Design review of the part built by this model. Coordinates are the model's own, in mm. Coordinates: 2 decimals unless noted, no trailing zeros. Write each loop counter-clockwise with the first axis right and the second up, starting at its lowest first coordinate (ties: lowest second). Pieces come first, ordered by that corner, then holes. Notation, with made-up numbers: (-14.75, 78.5) - (12.25, 78.5) arc R34 cw to (12.25, 111.5) - close; hole circle Ø8 at (61.5, -35.5). An arc over 180 degrees is marked (long way). Use a Markdown table: item, result.
from build123d import *

# Parameters (mm, degrees)
CROQUIS1_R              = 1.5
SALIENTE_EXTRUIR2_DEPTH = 2.5
CROQUIS2_R              = 2.5
CORTAR_EXTRUIR1_DEPTH   = 2.5
REDONDEO1_R             = 3


with BuildPart() as part:
    # Croquis1 → Saliente-Extruir2 (new body)
    with BuildSketch(Plane.XY):
        with BuildLine():
            Line((-71.814275766, 92), (-71.814275766, 5))
            ThreePointArc((-71.814275766, 5), (-70.349809672, 1.464466094), (-66.814275766, 0))
            Line((-66.814275766, 0), (89.815390375, 0))
            ThreePointArc((89.815390375, 0), (91.936710719, 0.878679656), (92.815390375, 3))
            Line((92.815390375, 3), (92.815390375, 94))
            ThreePointArc((92.815390375, 94), (91.936710719, 96.121320344), (89.815390375, 97))
            Line((89.815390375, 97), (-66.814275766, 97))
            ThreePointArc((-66.814275766, 97), (-70.349809672, 95.535533906), (-71.814275766, 92))
        make_face()
        with Locations((69.850202166, 89.208902584)):
            Circle(CROQUIS1_R, mode=Mode.SUBTRACT)
        with Locations((-49, 89)):
            Circle(CROQUIS1_R, mode=Mode.SUBTRACT)
        with Locations((-49, 8)):
            Circle(CROQUIS1_R, mode=Mode.SUBTRACT)
        with Locations((70.315390375, 8)):
            Circle(CROQUIS1_R, mode=Mode.SUBTRACT)
    extrude(amount=SALIENTE_EXTRUIR2_DEPTH)

    # Croquis2 → Cortar-Extruir1 (cut)
    with BuildSketch(Plane.XY.offset(2.5)):
        with Locations((60.731545651, 10.35024669)):
            Circle(CROQUIS2_R)
        with Locations((60.731545651, 87.35024669)):
            Circle(CROQUIS2_R)
        with Locations((-20.117590151, 10.35024669)):
            Circle(CROQUIS2_R)
        with Locations((-20.117590151, 87.35024669)):
            Circle(CROQUIS2_R)
    extrude(amount=-CORTAR_EXTRUIR1_DEPTH, mode=Mode.SUBTRACT)

    # Redondeo1
    # the kernel refuses this fillet: 3 mm, written as the material it takes off along each edge
    with BuildSketch(Plane(origin=(89.815390375, 3, 2.5), x_dir=(0, -1, 0), z_dir=(-1, 0, 0))) as redondeo1_piece_1:
        with BuildLine():
            CenterArc((0.041960108, -3), REDONDEO1_R, 9.594068227, 80.405931773)
            Line((3, -2.5), (3.059160798, -2.49))
            ThreePointArc((3.059160798, -2.49), (3.06, -1.25), (3.06, 0))
            Line((3.06, 0), (3, 0.06))
            Line((3, 0.06), (0.041960108, 0.06))
            Line((0.041960108, 0.06), (0.041960108, 0))
        make_face()
    revolve(axis=Axis((89.815390375, 3, 2.5), (0, 0, 1)), revolution_arc=90, mode=Mode.SUBTRACT)
    with BuildSketch(Plane(origin=(-66.814275766, 0, 2.5), x_dir=(0, 1, 0), z_dir=(1, 0, 0)), Plane(origin=(89.815390375, 97, 2.5), x_dir=(0, -1, 0), z_dir=(-1, 0, 0))) as redondeo1_piece_2:
        with BuildLine():
            CenterArc((2.958039892, -3), REDONDEO1_R, 90, 80.405931773)
            Line((0, -2.5), (-0.059160798, -2.49))
            ThreePointArc((-0.059160798, -2.49), (-0.06, -1.25), (-0.06, 0))
            Line((-0.06, 0), (0, 0.06))
            Line((0, 0.06), (2.958039892, 0.06))
            Line((2.958039892, 0.06), (2.958039892, 0))
        make_face()
    extrude(amount=156.629666142, mode=Mode.SUBTRACT)
    with BuildSketch(Plane(origin=(-66.814275766, 5, 2.5), x_dir=(-1, 0, 0), z_dir=(0, 1, 0))) as redondeo1_piece_3:
        with BuildLine():
            CenterArc((2.041960108, -3), REDONDEO1_R, 9.594068227, 80.405931773)
            Line((2.041960108, 0), (2.041960108, 0.06))
            Line((2.041960108, 0.06), (5, 0.06))
            Line((5, 0.06), (5.06, 0))
            ThreePointArc((5.06, 0), (5.06, -1.25), (5.059160798, -2.49))
            Line((5.059160798, -2.49), (5, -2.5))
        make_face()
    revolve(axis=Axis((-66.814275766, 5, 2.5), (0, 0, 1)), revolution_arc=90, mode=Mode.SUBTRACT)
    with BuildSketch(Plane(origin=(-71.814275766, 92, 2.5), x_dir=(0, 0, -1), z_dir=(0, -1, 0))) as redondeo1_piece_4:
        with BuildLine():
            CenterArc((3, 2.958039892), REDONDEO1_R, 180, 80.405931773)
            Line((0, 2.958039892), (-0.06, 2.958039892))
            Line((-0.06, 2.958039892), (-0.06, 0))
            Line((-0.06, 0), (0, -0.06))
            ThreePointArc((0, -0.06), (1.25, -0.06), (2.49, -0.059160798))
            Line((2.49, -0.059160798), (2.5, 0))
        make_face()
    extrude(amount=87, mode=Mode.SUBTRACT)
    with BuildSketch(Plane(origin=(-66.814275766, 92, 2.5), x_dir=(0, 1, 0), z_dir=(1, 0, 0))) as redondeo1_piece_5:
        with BuildLine():
            CenterArc((2.041960108, -3), REDONDEO1_R, 9.594068227, 80.405931773)
            Line((2.041960108, 0), (2.041960108, 0.06))
            Line((2.041960108, 0.06), (5, 0.06))
            Line((5, 0.06), (5.06, 0))
            ThreePointArc((5.06, 0), (5.06, -1.25), (5.059160798, -2.49))
            Line((5.059160798, -2.49), (5, -2.5))
        make_face()
    revolve(axis=Axis((-66.814275766, 92, 2.5), (0, 0, 1)), revolution_arc=90, mode=Mode.SUBTRACT)
    with BuildSketch(Plane(origin=(89.815390375, 94, 2.5), x_dir=(1, 0, 0), z_dir=(0, -1, 0))) as redondeo1_piece_6:
        with BuildLine():
            CenterArc((0.041960108, -3), REDONDEO1_R, 9.594068227, 80.405931773)
            Line((3, -2.5), (3.059160798, -2.49))
            ThreePointArc((3.059160798, -2.49), (3.06, -1.25), (3.06, 0))
            Line((3.06, 0), (3, 0.06))
            Line((3, 0.06), (0.041960108, 0.06))
            Line((0.041960108, 0.06), (0.041960108, 0))
        make_face()
    revolve(axis=Axis((89.815390375, 94, 2.5), (0, 0, 1)), revolution_arc=90, mode=Mode.SUBTRACT)
    with BuildSketch(Plane(origin=(92.815390375, 3, 2.5), x_dir=(-1, 0, 0), z_dir=(0, 1, 0))) as redondeo1_piece_7:
        with BuildLine():
            CenterArc((2.958039892, -3), REDONDEO1_R, 90, 80.405931773)
            Line((0, -2.5), (-0.059160798, -2.49))
            ThreePointArc((-0.059160798, -2.49), (-0.06, -1.25), (-0.06, 0))
            Line((-0.06, 0), (0, 0.06))
            Line((0, 0.06), (2.958039892, 0.06))
            Line((2.958039892, 0.06), (2.958039892, 0))
        make_face()
    extrude(amount=91, mode=Mode.SUBTRACT)


solid = part.part
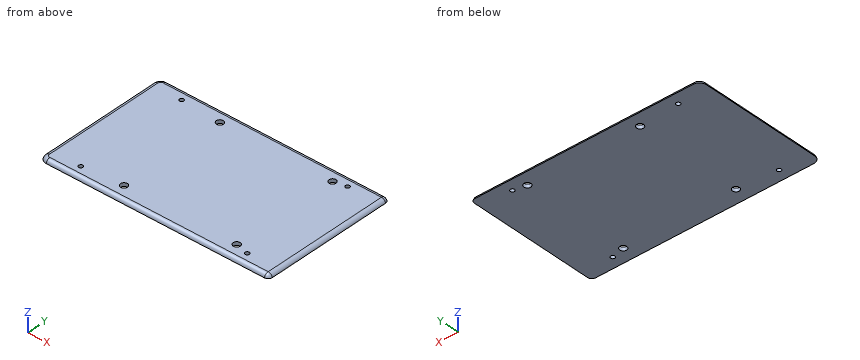
(1) For L1, parallel to Y at x = 60, z = 0.85; L2, parallel to Y at x = 59, z = 0.3; L3, parallel to X at y = 89, z = 1.95, list the stretches that pass through material, from the lowest coordinate up. Write a range as from..to.
Determined:
| item | result |
|---|---|
| L1 | 0.28..7.96, 12.74..84.96, 89.74..96.72 |
| L2 | 0.07..8.55, 12.15..85.55, 89.15..96.93 |
| L3 | -70.59..-50.5, -47.5..-22, -18.24..58.85, 62.61..68.36, 71.34..91.59 |
(2) For pin 1 (1.5 mm diameter, centred on x = -25, z = 1, fed in from -Y); pin 2 (1 mm diameter, centred on y = 41, z = 2, fed in from +X); pin 3 (1.5 mm diameter, centred on x = 50, z = 2, fed in from -Y), all flat-tipped, find the tip position at first contact; note any pin that passes through.
Determined:
| item | result |
|---|---|
| pin 1 | y = 0.05 |
| pin 2 | x = 92.09 |
| pin 3 | y = 0.52 |
(3) Take a section at B-B on x = -44.5. Write out the cut boundary in (y, z).
Determined:
| item | result |
|---|---|
| outline | (0, 0) - (97, 0) arc R3 ccw to (94.04, 2.5) - (2.96, 2.5) arc R3 ccw to start |
(4) Take a section at A-A on z = 1.8. State how many separate pieces and enclosed holes the cut face has, and give its area (3 significant figures).
Determined:
| item | result |
|---|---|
| separate pieces | 1 |
| enclosed holes | 8 |
| area | 15,300 mm2 |
